Work out the finished part from the listing and answer in its coordinate system (mm). A direction names the side the tool comes from. Coordinates: 2 decimals unless noted, no trailing zeros. Write each loop counter-clockwise with the first axis right and the second up, starting at its lowest first coordinate (ties: lowest second). Pieces come first, ordered by that corner, then holes. Notation, with made-up numbers: M -25,-28.5 L 0,-28.5 A33 cw 0,2.5 Z; hole C -1,-1.5 d7. An arc over 180 degrees is marked long. Use CSV: the item, a comma, the result in double quotes.
from build123d import *

# Parameters (mm, degrees)
BOSS_EXTRUDE1_DEPTH     = 10
CUT_EXTRUDE1_DEPTH      = 135.536240471
CUT_EXTRUDE1_DEPTH_BACK = 135.536240471
SKETCH3_R               = 4
FILLET1_R               = 10
BOSS_EXTRUDE2_OUTLINE_R = 5.5
BOSS_EXTRUDE2_DEPTH     = 40
BOSS_EXTRUDE2_START     = -5.5
BOSS_EXTRUDE2_2_DEPTH   = 11
SKETCH5_R               = 30
BOSS_EXTRUDE3_DEPTH     = 8
FILLET2_R               = 15
FILLET3_R               = 5


with BuildPart() as part:
    # Sketch2 → Boss-Extrude1 (new, symmetric)
    with BuildSketch(Plane.XY):
        with BuildLine():
            Line((0, 60), (10, 60))
            Line((10, 60), (10, 58))
            Line((10, 58), (0, 58))
            ThreePointArc((0, 58), (-58, 0), (0, -58))
            Line((0, -58), (10, -58))
            Line((10, -58), (10, -60))
            Line((10, -60), (0, -60))
            ThreePointArc((0, -60), (-60, 0), (0, 60))
        make_face()
    extrude(amount=BOSS_EXTRUDE1_DEPTH, both=True)

    # Sketch3 → Cut-Extrude1 (cut, two sides: drawn at the far end of the back side and taken through both)
    with BuildSketch(Plane(origin=(0, 60, 0), x_dir=(1, 0, 0), z_dir=(0, 1, 0)).offset(-CUT_EXTRUDE1_DEPTH_BACK)):
        with Locations(Location((0, 0, 0), (0, 0, 270))):
            Circle(SKETCH3_R)
    extrude(amount=CUT_EXTRUDE1_DEPTH + CUT_EXTRUDE1_DEPTH_BACK, mode=Mode.SUBTRACT)

    # Fillet1
    fillet1_edges = [part.edges().sort_by_distance(p)[0] for p in [
        (10, -59, -10),
        (10, -59, 10),
        (10, 59, -10),
        (10, 59, 10),
    ]]
    fillet(fillet1_edges, radius=FILLET1_R - 0.0001)  # a hair under: the kernel refuses the full size

    # Boss-Extrude2: read off the stored shape, not the designer's step
    # Boss-Extrude2 outline → Boss-Extrude2 (add)
    with BuildSketch(Plane.XZ.offset(60)):
        Circle(BOSS_EXTRUDE2_OUTLINE_R)
    extrude(amount=BOSS_EXTRUDE2_DEPTH)

    # Boss-Extrude2 2 outline → Boss-Extrude2 2 (add)
    with BuildSketch(Plane.XY.offset(BOSS_EXTRUDE2_START)):
        with BuildLine():
            Line((5, -59.799688591), (4.000851892, -59.866461263))
            ThreePointArc((4.000851892, -59.866461263), (2.001539936, -59.966606023), (0, -60))
            Line((0, -60), (5, -60))
            Line((5, -60), (5, -59.799688591))
        make_face()
    extrude(amount=BOSS_EXTRUDE2_2_DEPTH)

    # Sketch5 → Boss-Extrude3 (add)
    with BuildSketch(Plane.XZ.offset(100)):
        with Locations(Location((0, 0, 0), (0, 0, 270))):
            Circle(SKETCH5_R)
    extrude(amount=BOSS_EXTRUDE3_DEPTH)

    # Fillet2
    fillet2_edges = [part.edges().sort_by_distance(p)[0] for p in [
        (-5.5, -100, 0),
    ]]
    fillet(fillet2_edges, radius=FILLET2_R)

    # Fillet3
    fillet3_edges = [part.edges().sort_by_distance(p)[0] for p in [
        (0, -100, 30),
    ]]
    fillet(fillet3_edges, radius=FILLET3_R)


solid = part.part
Item 1: A tool of negligible diameter and unlimited length cuts with its end or side. For faces 1 (the face through (-59, 5, -10)), 2 (the face through (-1.19, -72.32, -5.37)), 3 (the face through (6.99, -59.01, -7.15)), 4 (the face through (6.99, -59.01, 7.15)), 5 (the face through (-59, 5, 10)), from which of +Z, -Z, +X, -X, +Y, -Y can it reach the whole face along a straight path? Write none if from no direction.
Answer:
face 1,"-Z, +X, -X, +Y"
face 2,"none"
face 3,"-Z, +X, +Y"
face 4,"+Z, +X, +Y"
face 5,"+Z, +X, -X, +Y"
Item 2: The part is cut by section D-D (y = -51). Write down the section's boundary in (x, z), then the cut area to 3 significant figures.
Answer:
outline,"M -31.61,-10 L -27.62,-10 L -27.62,10 L -31.61,10 Z"
area,"79.7 mm2"
Item 3: Given pin 1 (6 mm diameter, centred on y = -35, z = 12.5, fed in from -X); pin 2 (12 mm diameter, centred on x = -8.5, z = -6.5, fed in from +Y); pin 3 (4 mm diameter, centred on y = -12.5, z = -12.5, fed in from -X); pin 4 (6 mm diameter, centred on y = -48.5, z = -9.5, fed in from +X), each flat-ended and moving along its own axis, determine where each tip first touches the part or whether it passes through.
Answer:
pin 1,"stops at x = -49.88"
pin 2,"stops at y = 59.95"
pin 3,"passes through"
pin 4,"stops at x = -26.68"
Item 4: The part is cut by section C-C (y = -94.5). Write down the section's boundary in (x, z), then the cut area to 3 significant figures.
Answer:
outline,"C 0,0 d17.78"
area,"248 mm2"
Item 5: The part is cut by section B-B (x = -23). Count the separate pieces of the cut face and the enclosed holes in it, then the cut area to 3 significant figures.
Answer:
separate pieces,"3"
enclosed holes,"0"
area,"377 mm2"
Item 6: The part is cut by section A-A (y = 0). Write down the section's boundary in (x, z).
Answer:
outline,"M -60,-10 L -58,-10 L -58,10 L -60,10 Z"
Item 7: Consider probe 1 along Y at (x, z) = (-18, -4.5); probe 2 along Y at (x, z) = (1, 7.5); probe 3 along Z at (x, y) = (0, -59.2). Determine where each line is inside the solid, lowest interval first.
Answer:
probe 1,"y = -108 to -99.87, -57.24 to -55.14, 55.14 to 57.24"
probe 2,"y = -108 to -92.6, -60 to -58, 58 to 60"
probe 3,"z = -10 to -4, 4 to 10"
Item 8: For a pull along Y with two mould halves and no side action, classify faces 6 (the face through (1.58, -59.98, -0.06)), 7 (the face through (1.32, -106.48, 29.97)), 8 (the face through (5, 58, 0)) as released by +Y, released by -Y, zero draft, split by the parting line, or undercut.
Answer:
face 6,"released by +Y"
face 7,"zero draft"
face 8,"undercut"
